Could you check a few things on this model? Use its own coordinates, in mm. A direction names the side the tool comes from. Coordinates: 2 decimals unless noted, no trailing zeros. Write each loop counter-clockwise with the first axis right and the second up, starting at its lowest first coordinate (ties: lowest second). Pieces come first, ordered by that corner, then holes.
```python
from build123d import *

# Parameters (mm, degrees)
SALIENTE_EXTRUIR1_DEPTH           = 23
CROQUIS2_W                        = 34
CROQUIS2_H                        = 6.2
CORTAR_EXTRUIR1_DEPTH             = 6.2
CROQUIS3_W                        = 21.5
CROQUIS3_H                        = 0.3
CORTAR_EXTRUIR2_DEPTH             = 6.2
CORTAR_EXTRUIR3_REACH             = 18.8
CROQUIS4_R                        = 1.6
CORTAR_EXTRUIR4_DEPTH             = 9.8
CORTAR_EXTRUIR5_REACH             = 8.5
CROQUIS6_R                        = 1.6
CORTAR_EXTRUIR6_REACH             = 24.5
CROQUIS7_R                        = 1.6
SALIENTE_EXTRUIR2_DEPTH           = 23
CORTAR_EXTRUIR7_DEPTH             = 4
CORTAR_EXTRUIR7_DIRECTION_2_REACH = 18.5
CORTAR_EXTRUIR8_DEPTH             = 3


with BuildPart() as part:
    # Croquis1 → Saliente-Extruir1 (new body)
    with BuildSketch(Plane.XY):
        Polygon((0, 0), (9, 0), (9, 4), (24, 4), (24, 22.5), (-10, 22.5), (-10, 16), (11.5, 16), (11.5, 6), (0, 6), align=None)
    extrude(amount=SALIENTE_EXTRUIR1_DEPTH)

    # Croquis2 → Cortar-Extruir1 (cut)
    with BuildSketch(Plane.XY.offset(23)):
        with Locations((7, 19.4)):
            Rectangle(CROQUIS2_W, CROQUIS2_H)
    extrude(amount=-CORTAR_EXTRUIR1_DEPTH, mode=Mode.SUBTRACT)

    # Croquis3 → Cortar-Extruir2 (cut)
    with BuildSketch(Plane.XY.offset(23)):
        with Locations((0.75, 16.15)):
            Rectangle(CROQUIS3_W, CROQUIS3_H)
    extrude(amount=-CORTAR_EXTRUIR2_DEPTH, mode=Mode.SUBTRACT)

    # Croquis4 → Cortar-Extruir3 (cut, up to next)
    with BuildSketch(Plane.XY.offset(16.8), mode=Mode.PRIVATE) as cortar_extruir3_sk1:
        with Locations((-1.34, 19.4)):
            Circle(CROQUIS4_R)
    cortar_extruir3_tool1 = extrude(cortar_extruir3_sk1.sketch, amount=-CORTAR_EXTRUIR3_REACH, mode=Mode.PRIVATE) & part.part
    add(cortar_extruir3_tool1.solids().sort_by_distance((-1.34, 19.4, 16.8))[0], mode=Mode.SUBTRACT)

    # Croquis5 → Cortar-Extruir4 (cut)
    with BuildSketch(Plane(origin=(0, 0, 0), x_dir=(-1, 0, 0), z_dir=(0, 0, -1))):
        Polygon((-1.950896534, 19.4), (-0.305448267, 16.55), (2.985448267, 16.55), (4.630896534, 19.4), (2.985448267, 22.25), (-0.305448267, 22.25), align=None)
    extrude(amount=-CORTAR_EXTRUIR4_DEPTH, mode=Mode.SUBTRACT)

    # Croquis6 → Cortar-Extruir5 (cut, up to next)
    with BuildSketch(Plane.XZ.offset(-16), mode=Mode.PRIVATE) as cortar_extruir5_sk1:
        with Locations((6.73, 2.2)):
            Circle(CROQUIS6_R)
    cortar_extruir5_tool1 = extrude(cortar_extruir5_sk1.sketch, amount=-CORTAR_EXTRUIR5_REACH, mode=Mode.PRIVATE) & part.part
    add(cortar_extruir5_tool1.solids().sort_by_distance((6.73, 16, 2.2))[0], mode=Mode.SUBTRACT)

    # Croquis7 → Cortar-Extruir6 (cut, up to next)
    with BuildSketch(Plane.XZ, mode=Mode.PRIVATE) as cortar_extruir6_sk1:
        with Locations((4.95, 3.3)):
            Circle(CROQUIS7_R)
    cortar_extruir6_tool1 = extrude(cortar_extruir6_sk1.sketch, amount=-CORTAR_EXTRUIR6_REACH, mode=Mode.PRIVATE) & part.part
    add(cortar_extruir6_tool1.solids().sort_by_distance((4.95, 0, 3.3))[0], mode=Mode.SUBTRACT)

    # Croquis10 → Saliente-Extruir2 (add)
    with BuildSketch(Plane(origin=(0, 0, 0), x_dir=(-1, 0, 0), z_dir=(0, 0, -1))):
        Polygon((-11.5, 6), (-5.5, 6), (-11.5, 12), align=None)
    extrude(amount=-SALIENTE_EXTRUIR2_DEPTH)

    # Croquis8 → Cortar-Extruir7 (cut)
    with BuildSketch(Plane(origin=(0, 6, 0), x_dir=(1, 0, 0), z_dir=(0, 1, 0))):
        Polygon((1.659103466, -3.3), (3.304551733, -6.15), (6.595448267, -6.15), (8.240896534, -3.3), (6.595448267, -0.45), (3.304551733, -0.45), align=None)
    extrude(amount=-CORTAR_EXTRUIR7_DEPTH, mode=Mode.SUBTRACT)

    # Croquis8 → Cortar-Extruir7 direction 2 (cut, up to next)
    with BuildSketch(Plane(origin=(0, 6, 0), x_dir=(1, 0, 0), z_dir=(0, 1, 0)), mode=Mode.PRIVATE) as cortar_extruir7_direction_2_sk1:
        Polygon((1.659103466, -3.3), (3.304551733, -6.15), (6.595448267, -6.15), (8.240896534, -3.3), (6.595448267, -0.45), (3.304551733, -0.45), align=None)
    cortar_extruir7_direction_2_tool1 = extrude(cortar_extruir7_direction_2_sk1.sketch, amount=CORTAR_EXTRUIR7_DIRECTION_2_REACH, mode=Mode.PRIVATE) & part.part
    add(cortar_extruir7_direction_2_tool1.solids().sort_by_distance((4.95, 6, 3.3))[0], mode=Mode.SUBTRACT)

    # Croquis9 → Cortar-Extruir8 (cut)
    with BuildSketch(Plane(origin=(0, 22.5, 0), x_dir=(1, 0, 0), z_dir=(0, 1, 0))):
        Polygon((3.439103466, -2.2), (5.084551733, -5.05), (8.375448267, -5.05), (10.020896534, -2.2), (8.375448267, 0.65), (5.084551733, 0.65), align=None)
    extrude(amount=-CORTAR_EXTRUIR8_DEPTH, mode=Mode.SUBTRACT)


solid = part.part
```
Item 1: Which directions (+Z, -Z, +X, -X, +Y, -Y) give clear straight access to the entire face, cutting with the end or side of a thin tool? Please do faces 1 (the flat face through (6, 19.5, 4)), 2 (the flat face through (7, 21, 5.05)), 3 (the flat face through (1, 16, 8)).
Item 2: Will these pins go through, and if not, where does the flat tip stop? pin 1 Ø3 at (x, z) = (16.5, 19) entering from +Y; pin 2 Ø5 at (x, y) = (2.5, 19) entering from +Z; pin 3 Ø4.5 at (y, z) = (1.5, 7.5) entering from +X.
Item 3: I want a section at B-B, the plane z = 6.75. List the corners of the cut face in (x, y) for me.
Item 4: I want a section at C-C, the plane y = 2.75. List the corners of the cut face in (x, z) for me, then the cut area to 3 significant figures.
Item 5: I want a section at A-A, the plane x = -1.34. List the corners of the cut face in (y, z) for me.
Item 6: If we mould it in two halves opening along Y, with no side actions, what happens to faces 4 (the flat face through (7, 19, 16.8)), 5 (the flat face through (18, 16.3, 20)), 6 (the flat face through (-3.8, 17.96, 4.83))? For each: released by +Y, released by -Y, zero draft, split by the parting line, or undercut.
Item 7: I want a section at D-D, the plane z = 20.75. List the corners of the cut face in (x, y) for me.
Item 8: If I drill on line 1 along Z through (x, y) = (4.95, 0.75); line 2 along Y through (x, z) = (2.5, 6.25); line 3 along Z through (x, y) = (6.73, 17.2), over which ranges is the centre line in solid material (lowest first)?
Taken from the geometry:
1. face 1: +Y
1. face 2: -Z, +Y
1. face 3: +Z, -Z, -X
2. pin 1: stops at y = 16.3
2. pin 2: stops at z = 16.8
2. pin 3: stops at x = 9
3. outline: (-10, 16) - (11.5, 16) - (11.5, 12) - (5.5, 6) - (0, 6) - (0, 0) - (9, 0) - (9, 4) - (24, 4) - (24, 22.5) - (-10, 22.5) - close; hole (-4.63, 19.4) - (-2.99, 16.55) - (0.31, 16.55) - (1.95, 19.4) - (0.31, 22.25) - (-2.99, 22.25) - close
4. outline: (0, 0) - (9, 0) - (9, 23) - (0, 23) - close; hole (1.66, 3.3) - (3.3, 0.45) - (6.6, 0.45) - (8.24, 3.3) - (6.6, 6.15) - (3.3, 6.15) - close
4. area: 179 mm2
5. outline: (16, 0) - (16.55, 0) - (16.55, 9.8) - (17.8, 9.8) - (17.8, 16.8) - (16, 16.8) - close; (21, 9.8) - (22.25, 9.8) - (22.25, 0) - (22.5, 0) - (22.5, 16.8) - (21, 16.8) - close
6. face 4: zero draft
6. face 5: released by +Y
6. face 6: undercut
7. outline: (0, 0) - (9, 0) - (9, 4) - (24, 4) - (24, 16.3) - (11.5, 16.3) - (11.5, 12) - (5.5, 6) - (0, 6) - close
8. line 1: z = 0 to 1.7, 4.9 to 23
8. line 2: y = 0 to 6, 16 to 22.5
8. line 3: z = 0 to 0.6, 3.8 to 16.8
